Read the model definition and answer for the solid it produces. Units are mm, in the model's axes. A direction names the side the tool comes from. Round coordinates to 2 decimals unless told otherwise and drop trailing zeros. Order: outer loops, then holes, each group sorted by start corner. A loop starts at its lowest first (then second) coordinate and runs counter-clockwise, first axis right, second up. Notation, with made-up numbers: (78.5, 20) -> (91.5, 20) arc R4 cw to (91.5, 24) -> close; hole circle Ø6 at (-0.75, 54). An arc over 180 degrees is marked (long way). Use a Markdown table: item, result. Add a question column.
1. Section C-C, the plane x = 11.25 is taken. Give the vertices of the cut face in (y, z), then the cut area to 3 significant figures.
2. Section B-B, the plane x = 0 is taken. Give the vertices of the cut face in (y, z).
3. Consider L1, parallel to X at y = 25, z = 3.9; L2, parallel to Y at x = 0, z = 3.55; L3, parallel to Y at x = 11.5, z = 24.5. Determine where each line is inside the solid, lowest interval first. Write a range as [from, to].
4. Given pin 1 (9.5 mm diameter, centred on x = 0, z = 20, fed in from +Y); pin 2 (6 mm diameter, centred on x = -2, z = 20.5, fed in from -Y); pin 3 (5 mm diameter, centred on x = 2.5, y = 22.5, fed in from +Z), each flat-ended and moving along its own axis, determine where each tip first touches the part or whether it passes through.
5. Section D-D, the plane z = 27 is taken. Give the vertices of the cut face in (x, y).
6. Section A-A, the plane z = 20 is taken. Give the vertices of the cut face in (x, y).
7. For faces 5 (the face through (15, 4, 16)), 6 (the face through (-4, 23, 5)), determine the directions among +Z, -Z, +X, -X, +Y, -Y from which every point of the face is accessible in a straight line to the end or side of a thin tool.
8. The mould has two halves that part along Z. Classify faces 1 (the face through (0, 2, 41)), 2 (the face through (0, 20, 0)), 3 (the face through (-15, 4, 16)), 4 (the face through (0, 2, 23)): +Z half, -Z half, draft (parallel to the pull), parting line (faces both ways), or undercut.
```python
from build123d import *

# Parameters (mm, degrees)
SKETCH_1_W          = 30
SKETCH_1_H          = 50
EXTRUDE_1_DEPTH     = 5
SKETCH_2_W          = 30
SKETCH_2_H          = 40
EXTRUDE_2_DEPTH     = 5
SKETCH_3_R          = 3
CUT_EXTRUDE_1_DEPTH = 66.76473219
SKETCH_4_R          = 3
CUT_EXTRUDE_2_DEPTH = 66.76473219


with BuildPart() as part:
    # 草图1 → 凸台-拉伸1 (new body)
    with BuildSketch(Plane(origin=(0, 0, 0), x_dir=(1, 0, 0), z_dir=(0, 1, 0))):
        with Locations((0, -25)):
            Rectangle(SKETCH_1_W, SKETCH_1_H)
    extrude(amount=EXTRUDE_1_DEPTH)

    # 草图2 → 凸台-拉伸2 (add)
    with BuildSketch(Plane.XY):
        with Locations((0, 20)):
            Rectangle(SKETCH_2_W, SKETCH_2_H)
    extrude(amount=EXTRUDE_2_DEPTH)

    # 草图3 → 切除-拉伸1 (cut, through all)
    with BuildSketch(Plane(origin=(0, 0, 0), x_dir=(1, 0, 0), z_dir=(0, 1, 0))):
        with Locations(Location((0, -20, 0), (0, 0, 90))):
            Circle(SKETCH_3_R)
        with Locations(Location((0, -38, 0), (0, 0, 90))):
            Circle(SKETCH_3_R)
    extrude(amount=CUT_EXTRUDE_1_DEPTH, mode=Mode.SUBTRACT)

    # 草图4 → 切除-拉伸2 (cut, through all)
    with BuildSketch(Plane.XY):
        with Locations((0, 25)):
            Circle(SKETCH_4_R)
    extrude(amount=CUT_EXTRUDE_2_DEPTH, mode=Mode.SUBTRACT)


solid = part.part
```
Verdict:
| question | item | result |
|---|---|---|
| 1 | outline | (0, 0) -> (40, 0) -> (40, 5) -> (5, 5) -> (5, 50) -> (0, 50) -> close |
| 1 | area | 425 mm2 |
| 2 | outline | (0, 0) -> (22, 0) -> (22, 5) -> (5, 5) -> (5, 17) -> (0, 17) -> close; (0, 23) -> (5, 23) -> (5, 35) -> (0, 35) -> close; (0, 41) -> (5, 41) -> (5, 50) -> (0, 50) -> close; (28, 0) -> (40, 0) -> (40, 5) -> (28, 5) -> close |
| 3 | L1 | x = [-15, -3], [3, 15] |
| 3 | L2 | y = [0, 22], [28, 40] |
| 3 | L3 | y = [0, 5] |
| 4 | pin 1 | stops at y = 5 |
| 4 | pin 2 | stops at y = 0 |
| 4 | pin 3 | stops at z = 5 |
| 5 | outline | (-15, 0) -> (15, 0) -> (15, 5) -> (-15, 5) -> close |
| 6 | outline | (-15, 0) -> (-3, 0) -> (-3, 5) -> (-15, 5) -> close; (3, 0) -> (15, 0) -> (15, 5) -> (3, 5) -> close |
| 7 | face 5 | +Z, -Z, +X, +Y, -Y |
| 7 | face 6 | +Z, +X, -X, +Y |
| 8 | face 1 | undercut |
| 8 | face 2 | -Z half |
| 8 | face 3 | draft |
| 8 | face 4 | undercut |
